Could you check a few things on this model? Use its own coordinates, in mm. A direction names the side the tool comes from. Round coordinates to 2 decimals unless told otherwise and drop trailing zeros. Loops run counter-clockwise (first coordinate to the right, second up) from the corner with the lowest first, then second, coordinate; pieces in that order, holes last. Notation, with made-up numbers: (17.25, 24) -> (28.25, 24) arc R15 ccw to (28.25, 45) -> close; hole circle Ø9 at (74, -30.75). An arc over 180 degrees is marked (long way). One line per item, written item: value.
```python
from build123d import *

# Parameters (mm, degrees)
F2_DEPTH = 762
F3_DEPTH = 1219.2
F1_R     = 152.4
F4_DEPTH = 838.2
F5_DEPTH = 889
F6_W     = 1066.8
F6_H     = 508
F7_DEPTH = 2270.76
F8_R     = 152.4


with BuildPart() as f2:
    # F1 (on Front) → F2 (new body)
    with BuildSketch(Plane.XZ):
        with BuildLine():
            Line((355.6, 254), (1168.4, 254))
            ThreePointArc((1168.4, 254), (891.1208831509, 488.1832892436), (787.4, 835.9871132594))
            Line((787.4, 835.9871132594), (787.4, 1219.2))
            Line((787.4, 1219.2), (0, 1219.2))
            Line((0, 1219.2), (-787.4, 1219.2))
            Line((-787.4, 1219.2), (-787.4, 835.9871132594))
            ThreePointArc((-787.4, 835.9871132594), (-891.1208831509, 488.1832892436), (-1168.4, 254))
            Line((-1168.4, 254), (-355.6, 254))
            Line((-355.6, 254), (-355.6, 381))
            Line((-355.6, 381), (-355.6, 736.6))
            ThreePointArc((-355.6, 736.6), (0, 1092.2), (355.6, 736.6))
            Line((355.6, 736.6), (355.6, 381))
            Line((355.6, 381), (355.6, 254))
        make_face()
    extrude(amount=F2_DEPTH)

    # F1 (on Front) → F3 (join)
    with BuildSketch(Plane.XZ):
        Polygon((-1168.4, 0), (0, 0), (1168.4, 0), (1168.4, 254), (355.6, 254), (0, 254), (-355.6, 254), (-1168.4, 254), align=None)
    extrude(amount=F3_DEPTH)

    # F1 (on Front) → F4 (join)
    with BuildSketch(Plane.XZ):
        with BuildLine():
            ThreePointArc((1.7647e-06, 381), (251.4471720139, 485.152829234), (355.6, 736.6))
            ThreePointArc((355.6, 736.6), (0, 1092.2), (-355.6, 736.6))
            ThreePointArc((-355.6, 736.6), (-251.447170766, 485.1528279861), (1.7647e-06, 381))
        make_face()
        with Locations((0, 736.6)):
            Circle(F1_R, mode=Mode.SUBTRACT)
        with BuildLine():
            Line((-355.6, 736.6), (-355.6, 381))
            Line((-355.6, 381), (1.7647e-06, 381))
            ThreePointArc((1.7647e-06, 381), (-251.447170766, 485.1528279861), (-355.6, 736.6))
        make_face()
        with BuildLine():
            Line((1.7647e-06, 381), (355.6, 381))
            Line((355.6, 381), (355.6, 736.6))
            ThreePointArc((355.6, 736.6), (251.4471720139, 485.152829234), (1.7647e-06, 381))
        make_face()
    extrude(amount=F4_DEPTH)

    # F1 (on Front) → F5 (join)
    with BuildSketch(Plane.XZ):
        Polygon((0, 254), (355.6, 254), (355.6, 381), (1.7647e-06, 381), (-355.6, 381), (-355.6, 254), align=None)
    extrude(amount=F5_DEPTH)

    # F6 (on face) → F7 (cut)
    with BuildSketch(Plane.XY.offset(1219.2)):
        with Locations((0, -254)):
            Rectangle(F6_W, F6_H)
    extrude(amount=-F7_DEPTH, mode=Mode.SUBTRACT)

    # F8
    f8_edges = [f2.edges().sort_by_distance(p)[0] for p in [
        (1168.4, -1219.2, 127),
        (-1168.4, -1219.2, 127),
    ]]
    fillet(f8_edges, radius=F8_R)


solid = f2.part
```
Item 1: If we mould it in two halves opening along X, with no side actions, what happens to faces 1 (the face through (5, -863, 381)), 2 (the face through (533.4, -258, 618)), 3 (the face through (-355.6, -810, 445))? For each: released by +X, released by -X, zero draft, split by the parting line, or undercut.
Output:
face 1: zero draft
face 2: undercut
face 3: released by -X
Item 2: If we section it at A-A on y = -236: List the corners of the cut face in (x, z) for me.
Output:
outline: (-1168.4, 0) -> (-533.4, 0) -> (-533.4, 1219.2) -> (-787.4, 1219.2) -> (-787.4, 835.99) arc R635 cw to (-1168.4, 254) -> close; (533.4, 0) -> (1168.4, 0) -> (1168.4, 254) arc R635 cw to (787.4, 835.99) -> (787.4, 1219.2) -> (533.4, 1219.2) -> close
Item 3: If we section it at B-B on x = 0: List the corners of the cut face in (y, z) for me, plus the area to 3 significant figures.
Output:
outline: (-1219.2, 0) -> (-508, 0) -> (-508, 584.2) -> (-838.2, 584.2) -> (-838.2, 381) -> (-889, 381) -> (-889, 254) -> (-1219.2, 254) -> close; (-838.2, 889) -> (-508, 889) -> (-508, 1219.2) -> (-762, 1219.2) -> (-762, 1092.2) -> (-838.2, 1092.2) -> close
area: 395,000 mm²
Item 4: I need wall thicknesses on line 1 (Z direction, x = 0, y = -668.5); line 2 (X direction, y = -286.5, z = 1089.5); line 3 (X direction, y = -387, z = 235). Which ranges of each line are inside material? Lowest first, please. Write a range as from..to.
Output:
line 1: z = 0..584.2, 889..1219.2
line 2: x = -787.4..-533.4, 533.4..787.4
line 3: x = -1168.4..-533.4, 533.4..1168.4
Item 5: If we section it at C-C on z = 675: List the corners of the cut face in (x, y) for me.
Output:
outline: (-808.15, -762) -> (-355.6, -762) -> (-355.6, -838.2) -> (-139.4, -838.2) -> (-139.4, -508) -> (-533.4, -508) -> (-533.4, 0) -> (-808.15, 0) -> close; (139.4, -838.2) -> (355.6, -838.2) -> (355.6, -762) -> (808.15, -762) -> (808.15, 0) -> (533.4, 0) -> (533.4, -508) -> (139.4, -508) -> close
Item 6: Will these pins go through, and if not, where does the flat tip stop? pin 1 Ø5 at (x, z) = (320.5, 734) entering from -Y; pin 2 Ø1 at (y, z) = (-610, 771) entering from +X; pin 3 Ø15 at (x, y) = (-4.5, -854.5) entering from +Z.
Output:
pin 1: stops at y = -838.2
pin 2: stops at x = 790.79
pin 3: stops at z = 381
Item 7: If we section it at D-D on z = 167.5: List the corners of the cut face in (x, y) for me, plus the area to 3 significant figures.
Output:
outline: (-1168.4, -1066.8) arc R152.4 ccw to (-1016, -1219.2) -> (1016, -1219.2) arc R152.4 ccw to (1168.4, -1066.8) -> (1168.4, 0) -> (533.4, 0) -> (533.4, -508) -> (-533.4, -508) -> (-533.4, 0) -> (-1168.4, 0) -> close
area: 2,300,000 mm²
Item 8: For faces 4 (the face through (-5, -889, 318)), 5 (the face through (787.4, -376, 1025)), 6 (the face through (-16, -737, 0)), 7 (the face through (-126, -508, 618)), 8 (the face through (7.819, -799.567, 1092.114)), which set-ups out of +Z, -Z, +X, -X, +Y, -Y let a thin tool reach every point of the face, with its end or its side?
Output:
face 4: +Z, +X, -X, -Y
face 5: +Z, +X, +Y, -Y
face 6: -Z, +X, -X, +Y, -Y
face 7: +Z, -Z, +Y
face 8: +Z, -Y
